Read the model definition and answer for the solid it produces. Units are mm, in the model's axes. Face numbers are marked on the shaded views. Coordinates: 2 decimals unless noted, no trailing zeros. Write each loop counter-clockwise with the first axis right and the second up, starting at its lowest first coordinate (ties: lowest second). Pieces come first, ordered by that corner, then holes. Notation, with made-up numbers: (-16, -34.5) - (19, -34.5) arc R18 ccw to (19, -29.5) - close; hole circle Ø6 at (-5, 40.5). An arc over 180 degrees is marked (long way). Use a Markdown table: item, result.
from build123d import *

# Parameters (mm, degrees)
RESSALTO_EXTRUS_O1_DEPTH     = 3
PERFIL_CORTE_W               = 23
PERFIL_CORTE_H               = 12.4
CORTE_PRINCIPAL_DEPTH        = 112.01996056
ESBO_O7_W                    = 12
ESBO_O7_H                    = 3
ESBO_O7_W_2                  = 17.5
CORTE_EXTRUS_O3_DEPTH        = 70.828040064
FURO_DE_DI_METRO_2_6_2_6_1_D = 2.6


with BuildPart() as part:
    # Base Perfil → Ressalto-extrusão1 (new body)
    with BuildSketch(Plane(origin=(0, 0, 0), x_dir=(1, 0, 0), z_dir=(0, 1, 0))):
        with BuildLine():
            Line((-17.5, 12.5), (14.5, 12.5))
            ThreePointArc((14.5, 12.5), (17.769603256, 10.248877314), (16.833333333, 6.391254026))
            ThreePointArc((16.833333333, 6.391254026), (16.587129071, 6.054146324), (16.5, 5.645898034))
            Line((16.5, 5.645898034), (16.5, -5.645898034))
            ThreePointArc((16.5, -5.645898034), (16.587129071, -6.054146324), (16.833333333, -6.391254026))
            ThreePointArc((16.833333333, -6.391254026), (17.769603256, -10.248877314), (14.5, -12.5))
            Line((14.5, -12.5), (-17.5, -12.5))
            Line((-17.5, -12.5), (-17.5, 12.5))
        make_face()
    extrude(amount=RESSALTO_EXTRUS_O1_DEPTH)

    # Perfil Corte → Corte Principal (cut, through all)
    with BuildSketch(Plane(origin=(-89.30915689, 3, 15.805061213), x_dir=(1, 0, 0), z_dir=(0, 1, 0))):
        with Locations((89.98915689, 15.805061213)):
            Rectangle(PERFIL_CORTE_W, PERFIL_CORTE_H)
    extrude(amount=-CORTE_PRINCIPAL_DEPTH, mode=Mode.SUBTRACT)

    # Esboço7 → Corte-extrusão3 (cut, through all)
    with BuildSketch(Plane(origin=(-37.630551407, 3, 29.597469394), x_dir=(1, 0, 0), z_dir=(0, 1, 0))):
        with Locations((38.310551407, 37.297469394)):
            Rectangle(ESBO_O7_W, ESBO_O7_H)
        with Locations((38.310551407, 21.897469394)):
            Rectangle(ESBO_O7_W_2, ESBO_O7_H)
    extrude(amount=-CORTE_EXTRUS_O3_DEPTH, mode=Mode.SUBTRACT)

    # Furo de diâmetro Ø2.6 (2.6)1 (through all)
    with Locations(Plane(origin=(0, 3, 0), x_dir=(1, 0, 0), z_dir=(0, 1, 0))):
        with Locations((-14.5, 9), (-14.5, -9), (14.5, 9), (14.5, -9)):
            Hole(FURO_DE_DI_METRO_2_6_2_6_1_D / 2)


solid = part.part
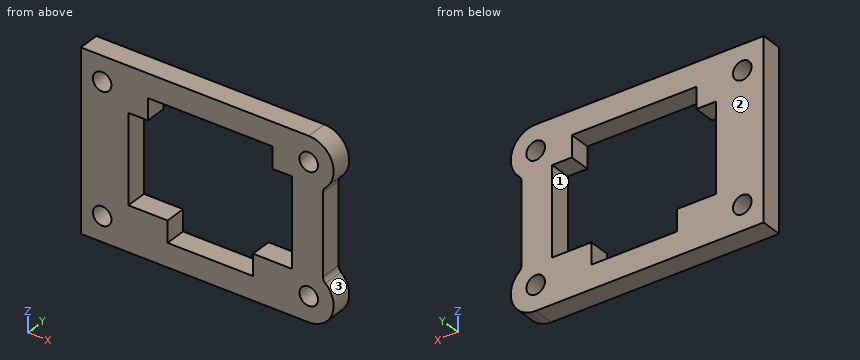
(1) A cutting plane is placed at A-A, the plane z = 1.75. Write down the section's boundary in (x, y).
Report:
| item | result |
|---|---|
| outline | (-17.5, 0) - (-10.82, 0) - (-10.82, 3) - (-17.5, 3) - close; (12.18, 0) - (16.5, 0) - (16.5, 3) - (12.18, 3) - close |
(2) A cutting plane is placed at B-B, the plane x = -14.5. Write down the section's boundary in (y, z).
Report:
| item | result |
|---|---|
| outline | (0, -12.5) - (3, -12.5) - (3, -10.3) - (0, -10.3) - close; (0, -7.7) - (3, -7.7) - (3, 7.7) - (0, 7.7) - close; (0, 10.3) - (3, 10.3) - (3, 12.5) - (0, 12.5) - close |
(3) The mould has two halves that part along Z. Classify the marked faces 1, 2 and 3: pulls with the +Z half, pulls with the -Z half, needs draft (parallel to the pull), parting line crosses it, or undercut.
Report:
| item | result |
|---|---|
| face 1 | undercut |
| face 2 | needs draft |
| face 3 | undercut |
(4) A cutting plane is placed at D-D, the plane x = 11. Write down the section's boundary in (y, z).
Report:
| item | result |
|---|---|
| outline | (0, -12.5) - (3, -12.5) - (3, -6.2) - (0, -6.2) - close; (0, 6.2) - (3, 6.2) - (3, 12.5) - (0, 12.5) - close |
(5) Each of these flat-tipped pins is pushed along its axis until it touches: P1, Ø1.5, axis at y = 2, z = -2.5, coming from the +X side; P2, Ø1.5, axis at y = 2, z = -7.5, coming from the +X side; P3, Ø4, axis at x = -14.5, z = 9, coming from the -Y side; P4, Ø0.9, axis at y = 1.5, z = 8, coming from the +X side. Where does it stop, or does it pass through?
Report:
| item | result |
|---|---|
| P1 | stops at x = 16.5 |
| P2 | stops at x = 17.92 |
| P3 | stops at y = 0 |
| P4 | stops at x = 17.96 |
(6) A cutting plane is placed at C-C, the plane y = 0.7. Write down the section's boundary in (x, z).
Report:
| item | result |
|---|---|
| outline | (-17.5, -12.5) - (14.5, -12.5) arc R3.5 ccw to (16.83, -6.39) arc R1 cw to (16.5, -5.65) - (16.5, 5.65) arc R1 cw to (16.83, 6.39) arc R3.5 ccw to (14.5, 12.5) - (-17.5, 12.5) - close; hole circle Ø2.6 at (-14.5, -9); hole circle Ø2.6 at (-14.5, 9); hole (-10.82, -6.2) - (-5.32, -6.2) - (-5.32, -9.2) - (6.68, -9.2) - (6.68, -6.2) - (12.18, -6.2) - (12.18, 6.2) - (9.43, 6.2) - (9.43, 9.2) - (-8.07, 9.2) - (-8.07, 6.2) - (-10.82, 6.2) - close; hole circle Ø2.6 at (14.5, -9); hole circle Ø2.6 at (14.5, 9) |
(7) Straight lines are drawn through the part: L1, parallel to X at y = 2.25, z = -9; L2, parallel to Z at x = 14.5, y = 2; L3, parallel to X at y = 1.3, z = 5.5. For each, find the intervals that lie inside material, in ascending order.
Report:
| item | result |
|---|---|
| L1 | x = -17.5 to -15.8, -13.2 to -5.32, 6.68 to 13.2, 15.8 to 18 |
| L2 | z = -12.5 to -10.3, -7.7 to 7.7, 10.3 to 12.5 |
| L3 | x = -17.5 to -10.82, 12.18 to 16.5 |
